Design review of the part built by this model. Coordinates are the model's own, in mm. Round coordinates to 2 decimals unless told otherwise and drop trailing zeros. Loops run counter-clockwise (first coordinate to the right, second up) from the corner with the lowest first, then second, coordinate; pieces in that order, holes last. Notation, with made-up numbers: M 64,20 L 112,20 A9 cw 112,37 Z; hole C 43.5,17 d4. An arc over 180 degrees is marked long. Use a Markdown table: item, result.
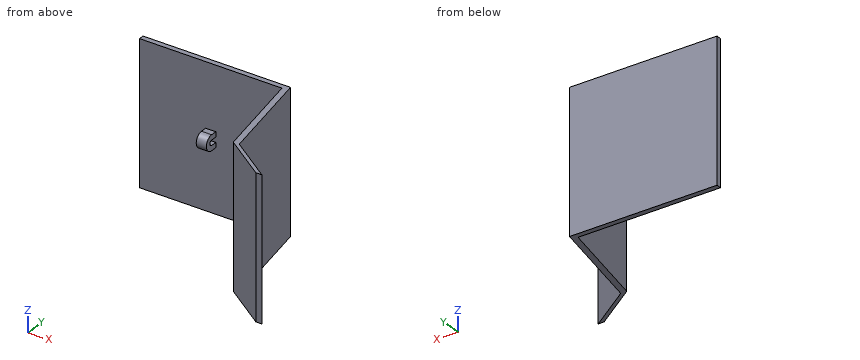
from build123d import *

# Parameters (mm, degrees)
SKETCH1_W           = 355.6
SKETCH1_H           = 355.6
BOSS_EXTRUDE1_DEPTH = 12.7
BOSS_EXTRUDE2_DEPTH = 12.7
BOSS_EXTRUDE4_DEPTH = 355.6


with BuildPart() as part:
    # Sketch1 → Boss-Extrude1 (new body)
    with BuildSketch(Plane(origin=(0, 0, 0), x_dir=(1, 0, 0), z_dir=(0, 1, 0))):
        with Locations((177.8, 177.8)):
            Rectangle(SKETCH1_W, SKETCH1_H)
    extrude(amount=BOSS_EXTRUDE1_DEPTH)

    # Sketch3 → Boss-Extrude2 (add, symmetric)
    with BuildSketch(Plane(origin=(177.8, 0, 0), x_dir=(0, 0, -1), z_dir=(1, 0, 0))):
        with BuildLine():
            Line((158.75, 0), (158.75, -15))
            ThreePointArc((158.75, -15), (177.8, -34.05), (196.85, -15))
            Line((196.85, -15), (196.85, 0))
            Line((196.85, 0), (184.15, 0))
            Line((184.15, 0), (184.15, -15))
            ThreePointArc((184.15, -15), (177.8, -21.35), (171.45, -15))
            Line((171.45, -15), (171.45, 0))
            Line((171.45, 0), (158.75, 0))
        make_face()
    extrude(amount=BOSS_EXTRUDE2_DEPTH, both=True)

    # Sketch6 → Boss-Extrude4 (add)
    with BuildSketch(Plane.XY):
        Polygon((368.3, 12.7), (412.406637127, -237.441169265), (521.231515241, -313.641169265), (506.292162586, -313.641169265), (397.467284472, -237.441169265), (355.6, 0), (355.6, 12.7), align=None)
    extrude(amount=-BOSS_EXTRUDE4_DEPTH)


solid = part.part
1. Wall thickness on line 1 along Y through (x, z) = (37.5, -15); line 2 along X through (y, z) = (-237.5, -263); line 3 along Y through (x, z) = (453, -140.5): over which ranges is each line inside the solid? List them lowest first. Write a range as from..to.
Check values:
| item | result |
|---|---|
| line 1 | y = 0..12.7 |
| line 2 | x = 397.55..412.49 |
| line 3 | y = -276.33..-265.86 |
2. Take a section at B-B on x = 183.5. Give the boundary of the cut face in (y, z), and give its area (3 significant figures).
Check values:
| item | result |
|---|---|
| outline | M -15,-196.85 L 0,-196.85 L 0,-355.6 L 12.7,-355.6 L 12.7,0 L 0,0 L 0,-158.75 L -15,-158.75 A19.05 ccw Z; hole M -15,-184.15 L 0,-184.15 L 0,-171.45 L -15,-171.45 A6.35 ccw Z |
| area | 5,400 mm² |
3. Take a section at A-A on z = -177.8. Give the boundary of the cut face in (x, y), and give its area (3 significant figures).
Check values:
| item | result |
|---|---|
| outline | M 0,0 L 355.6,0 L 397.47,-237.44 L 506.29,-313.64 L 521.23,-313.64 L 412.41,-237.44 L 368.3,12.7 L 0,12.7 Z; M 165.1,-34.05 L 190.5,-34.05 L 190.5,-21.35 L 165.1,-21.35 Z |
| area | 9,700 mm² |
4. Take a section at C-C on z = -41. Give the boundary of the cut face in (x, y).
Check values:
| item | result |
|---|---|
| outline | M 0,0 L 355.6,0 L 397.47,-237.44 L 506.29,-313.64 L 521.23,-313.64 L 412.41,-237.44 L 368.3,12.7 L 0,12.7 Z |
5. Insertion check: pin 1 (7.5 mm diameter, centred on x = 173.5, y = -10.5, fed in from +Z); pin 2 (3 mm diameter, centred on x = 333.5, z = -180.5, fed in from -Y); pin 3 (10 mm diameter, centred on y = -24, z = -171, fed in from +X). Each pin has a flat end and moves straight along its axis. Give the tip position at first contact, or say it passes through.
Check values:
| item | result |
|---|---|
| pin 1 | stops at z = -158.75 |
| pin 2 | stops at y = 0 |
| pin 3 | stops at x = 375.65 |
6. Take a section at D-D on y = -228.5. Give the boundary of the cut face in (x, z).
Check values:
| item | result |
|---|---|
| outline | M 395.89,-355.6 L 410.83,-355.6 L 410.83,0 L 395.89,0 Z |
